Work out the finished part from the listing and answer in its coordinate system (mm). A direction names the side the tool comes from. Give positions to 0.01 mm unless a question says otherwise; leave off trailing zeros. Write each loop counter-clockwise with the first axis right and the second up, starting at its lowest first coordinate (ties: lowest second). Pieces come first, ordered by that corner, then holes.
1) Straight lines are drawn through the part: probe 1 along X at (y, z) = (38, 20.75); probe 2 along Y at (x, z) = (50, 20.45); probe 3 along X at (y, z) = (4, 27.5). For each, find the intervals that lie inside material, in ascending order.
2) Find section A-A (y = 57.5). Determine the outline of the cut face in (x, z).
3) A tool of negligible diameter and unlimited length cuts with its end or side. For faces 1 (the face through (49, 57, 27)), 2 (the face through (63, 57, 24)), 3 (the face through (53, 57, 28)), 4 (the face through (52, 18, 28)), from which of +Z, -Z, +X, -X, +Y, -Y can it reach the whole face along a straight path? Write none if from no direction.
4) Find section B-B (x = 125). Determine the outline of the cut face in (y, z), plus the area to 3 significant figures.
5) Find section C-C (y = 24). Determine the outline of the cut face in (x, z).
6) Determine the mould class of faces 5 (the face through (52, 44, 28)), 6 (the face through (50.74, 36.58, 20.48)), 7 (the face through (62, 18, 28)), 8 (the face through (126.11, 11.54, 19.49)) for opening direction X: pulls with the +X half, pulls with the -X half, needs draft (parallel to the pull), parting line crosses it, or undercut.
7) Given pin 1 Ø2.5 at (x, z) = (62, 22) entering from -Y; pin 2 Ø1.1 at (x, z) = (68.5, 26.5) entering from +Y; pin 3 Ø5 at (x, y) = (124, 33.5) entering from +Z, each flat-ended and moving along its own axis, determine where each tip first touches the part or whether it passes through.
8) Find section D-D (x = 135). Determine the outline of the cut face in (y, z).
```python
from build123d import *

# Parameters (mm, degrees)
CYLINDER455_R     = 1.2
CYLINDER455_DEPTH = 4
CYLINDER454_R     = 1.2
CYLINDER454_DEPTH = 4
BOX307_W          = 4
BOX307_H          = 6
BOX307_DEPTH      = 1
BOX308_W          = 10.5
BOX308_H          = 6
BOX308_DEPTH      = 1
BOX306_W          = 4
BOX306_H          = 6
BOX306_DEPTH      = 1
BOX305_W          = 75
BOX305_H          = 62
BOX305_DEPTH      = 1
BOX304_W          = 25
BOX304_H          = 62
BOX304_DEPTH      = 1
BOX303_W          = 25
BOX303_H          = 82
BOX303_DEPTH      = 2
BOX302_W          = 25
BOX302_H          = 82
BOX302_DEPTH      = 3
FILLET108_R       = 2.99
CYLINDER349_R     = 1.6
CYLINDER349_DEPTH = 10
CYLINDER351_R     = 1.6
CYLINDER351_DEPTH = 10
CYLINDER350_R     = 1.6
CYLINDER350_DEPTH = 10
CYLINDER347_R     = 1.6
CYLINDER347_DEPTH = 10
CYLINDER353_R     = 1.6
CYLINDER353_DEPTH = 10
BOX241_W          = 19
BOX241_H          = 5
BOX241_DEPTH      = 5
BOX242_W          = 4
BOX242_H          = 5
BOX242_DEPTH      = 8
BOX243_W          = 1.8
BOX243_H          = 7
BOX243_DEPTH      = 11
BOX244_W          = 8
BOX244_H          = 5
BOX244_DEPTH      = 8
BOX245_W          = 24
BOX245_H          = 10
BOX245_DEPTH      = 15
FILLET095_R       = 6
CYLINDER352_R     = 1.6
CYLINDER352_DEPTH = 10
BOX240_W          = 19
BOX240_H          = 5
BOX240_DEPTH      = 5
BOX239_W          = 4
BOX239_H          = 5
BOX239_DEPTH      = 8
BOX238_W          = 1.8
BOX238_H          = 7
BOX238_DEPTH      = 11
BOX236_W          = 8
BOX236_H          = 5
BOX236_DEPTH      = 8
BOX237_W          = 24
BOX237_H          = 10
BOX237_DEPTH      = 15
FILLET094_R       = 6
CYLINDER355_R     = 1.6
CYLINDER355_DEPTH = 10
BOX247_W          = 10
BOX247_H          = 10
BOX247_DEPTH      = 12
CYLINDER354_R     = 1.6
CYLINDER354_DEPTH = 10
BOX246_W          = 10
BOX246_H          = 10
BOX246_DEPTH      = 12
BOX235_W          = 24
BOX235_H          = 42
BOX235_DEPTH      = 3
FILLET109_R       = 6


with BuildPart() as cylinder455:
    # Cylinder455 → Cylinder455 (new body)
    with BuildSketch(Plane(origin=(125, 50, 15), x_dir=(1, 0, 0), z_dir=(0, 0, 1))):
        Circle(CYLINDER455_R)
    extrude(amount=CYLINDER455_DEPTH)


with BuildPart() as fusion409:
    # Cylinder454 → Cylinder454 (new body)
    with BuildSketch(Plane(origin=(125, 12, 15), x_dir=(1, 0, 0), z_dir=(0, 0, 1))):
        Circle(CYLINDER454_R)
    extrude(amount=CYLINDER454_DEPTH)

    # Fusion409: union Cylinder455
    add(cylinder455.part)


with BuildPart() as fusion409_1:
    # Fusion409 placement: moved
    add(fusion409.part.moved(Location((0, 0, 1))))


with BuildPart() as cube378:
    # Box307 → Box307 (new body)
    with BuildSketch(Plane(origin=(69, 54, 19), x_dir=(1, 0, 0), z_dir=(0, 0, 1))):
        with Locations((2, 3)):
            Rectangle(BOX307_W, BOX307_H)
    extrude(amount=BOX307_DEPTH)


with BuildPart() as cube379:
    # Box308 → Box308 (new body)
    with BuildSketch(Plane(origin=(133.5, 28, 19), x_dir=(1, 0, 0), z_dir=(0, 0, 1))):
        with Locations((5.25, 3)):
            Rectangle(BOX308_W, BOX308_H)
    extrude(amount=BOX308_DEPTH)


with BuildPart() as fusion410:
    # Box306 → Box306 (new body)
    with BuildSketch(Plane(origin=(69, 2, 19), x_dir=(1, 0, 0), z_dir=(0, 0, 1))):
        with Locations((2, 3)):
            Rectangle(BOX306_W, BOX306_H)
    extrude(amount=BOX306_DEPTH)

    # Fusion408: union Cube378, Cube379
    add(cube378.part)
    add(cube379.part)

    # Fusion410: union Fusion409
    add(fusion409_1.part)


with BuildPart() as cut303:
    # Box305 → Box305 (new body)
    with BuildSketch(Plane(origin=(69, 0, 19), x_dir=(1, 0, 0), z_dir=(0, 0, 1))):
        with Locations((37.5, 31)):
            Rectangle(BOX305_W, BOX305_H)
    extrude(amount=BOX305_DEPTH)

    # Cut303: cut Fusion410
    add(fusion410.part, mode=Mode.SUBTRACT)


with BuildPart() as cube375:
    # Box304 → Box304 (new body)
    with BuildSketch(Plane(origin=(45, 0, 19), x_dir=(1, 0, 0), z_dir=(0, 0, 1))):
        with Locations((12.5, 31)):
            Rectangle(BOX304_W, BOX304_H)
    extrude(amount=BOX304_DEPTH)


with BuildPart() as cube374:
    # Box303 → Box303 (new body)
    with BuildSketch(Plane(origin=(45, -10, 17), x_dir=(1, 0, 0), z_dir=(0, 0, 1))):
        with Locations((12.5, 41)):
            Rectangle(BOX303_W, BOX303_H)
    extrude(amount=BOX303_DEPTH)


with BuildPart() as fusion411:
    # Box302 → Box302 (new body)
    with BuildSketch(Plane(origin=(45, -10, 17), x_dir=(1, 0, 0), z_dir=(0, 0, 1))):
        with Locations((12.5, 41)):
            Rectangle(BOX302_W, BOX302_H)
    extrude(amount=BOX302_DEPTH)

    # Fillet108
    fillet108_edges = [fusion411.edges().sort_by_distance(p)[0] for p in [
        (57.5, -10, 20),
        (57.5, 72, 20),
    ]]
    fillet(fillet108_edges, radius=FILLET108_R)

    # Cut301: cut Cube374
    add(cube374.part, mode=Mode.SUBTRACT)

    # Cut302: cut Cube375
    add(cube375.part, mode=Mode.SUBTRACT)

    # Fusion411: union Cut303
    add(cut303.part)


with BuildPart() as cylinder349:
    # Cylinder349 → Cylinder349 (new body)
    with BuildSketch(Plane(origin=(50, 24, 12), x_dir=(1, 0, 0), z_dir=(0, 0, 1))):
        Circle(CYLINDER349_R)
    extrude(amount=CYLINDER349_DEPTH)


with BuildPart() as cylinder351:
    # Cylinder351 → Cylinder351 (new body)
    with BuildSketch(Plane(origin=(64, 24, 12), x_dir=(1, 0, 0), z_dir=(0, 0, 1))):
        Circle(CYLINDER351_R)
    extrude(amount=CYLINDER351_DEPTH)


with BuildPart() as cylinder350:
    # Cylinder350 → Cylinder350 (new body)
    with BuildSketch(Plane(origin=(64, 38, 12), x_dir=(1, 0, 0), z_dir=(0, 0, 1))):
        Circle(CYLINDER350_R)
    extrude(amount=CYLINDER350_DEPTH)


with BuildPart() as fusion300:
    # Cylinder347 → Cylinder347 (new body)
    with BuildSketch(Plane(origin=(50, 38, 12), x_dir=(1, 0, 0), z_dir=(0, 0, 1))):
        Circle(CYLINDER347_R)
    extrude(amount=CYLINDER347_DEPTH)

    # Fusion300: union Cylinder349, Cylinder351, Cylinder350
    add(cylinder349.part)
    add(cylinder351.part)
    add(cylinder350.part)


with BuildPart() as cylinder353:
    # Cylinder353 → Cylinder353 (new body)
    with BuildSketch(Plane(origin=(57, 52, 30), x_dir=(1, 0, 0), z_dir=(0, -1, 0))):
        Circle(CYLINDER353_R)
    extrude(amount=CYLINDER353_DEPTH)


with BuildPart() as cube321:
    # Box241 → Box241 (new body)
    with BuildSketch(Plane(origin=(54, 44.5, 19), x_dir=(1, 0, 0), z_dir=(0, 0, 1))):
        with Locations((9.5, 2.5)):
            Rectangle(BOX241_W, BOX241_H)
    extrude(amount=BOX241_DEPTH)


with BuildPart() as cube322:
    # Box242 → Box242 (new body)
    with BuildSketch(Plane(origin=(54, 44.5, 19), x_dir=(1, 0, 0), z_dir=(0, 0, 1))):
        with Locations((2, 2.5)):
            Rectangle(BOX242_W, BOX242_H)
    extrude(amount=BOX242_DEPTH)


with BuildPart() as cube323:
    # Box243 → Box243 (new body)
    with BuildSketch(Plane(origin=(53, 43.5, 19), x_dir=(1, 0, 0), z_dir=(0, 0, 1))):
        with Locations((0.9, 3.5)):
            Rectangle(BOX243_W, BOX243_H)
    extrude(amount=BOX243_DEPTH)


with BuildPart() as cube324:
    # Box244 → Box244 (new body)
    with BuildSketch(Plane(origin=(45, 44.5, 19), x_dir=(1, 0, 0), z_dir=(0, 0, 1))):
        with Locations((4, 2.5)):
            Rectangle(BOX244_W, BOX244_H)
    extrude(amount=BOX244_DEPTH)


with BuildPart() as fillet095:
    # Box245 → Box245 (new body)
    with BuildSketch(Plane(origin=(45, 42, 19), x_dir=(1, 0, 0), z_dir=(0, 0, 1))):
        with Locations((12, 5)):
            Rectangle(BOX245_W, BOX245_H)
    extrude(amount=BOX245_DEPTH)

    # Cut250: cut Cube324
    add(cube324.part, mode=Mode.SUBTRACT)

    # Cut254: cut Cube323
    add(cube323.part, mode=Mode.SUBTRACT)

    # Cut253: cut Cube322
    add(cube322.part, mode=Mode.SUBTRACT)

    # Cut251: cut Cube321
    add(cube321.part, mode=Mode.SUBTRACT)

    # Cut252: cut Cylinder353
    add(cylinder353.part, mode=Mode.SUBTRACT)

    # Fillet095
    fillet095_edges = [fillet095.edges().sort_by_distance(p)[0] for p in [
        (45, 47, 34),
        (69, 47, 34),
    ]]
    fillet(fillet095_edges, radius=FILLET095_R)


with BuildPart() as fillet095_1:
    # Fillet095 placement: moved
    add(fillet095.part.moved(Location((0, 10, 0))))


with BuildPart() as cylinder352:
    # Cylinder352 → Cylinder352 (new body)
    with BuildSketch(Plane(origin=(57, 52, 30), x_dir=(1, 0, 0), z_dir=(0, -1, 0))):
        Circle(CYLINDER352_R)
    extrude(amount=CYLINDER352_DEPTH)


with BuildPart() as cube320:
    # Box240 → Box240 (new body)
    with BuildSketch(Plane(origin=(54, 44.5, 19), x_dir=(1, 0, 0), z_dir=(0, 0, 1))):
        with Locations((9.5, 2.5)):
            Rectangle(BOX240_W, BOX240_H)
    extrude(amount=BOX240_DEPTH)


with BuildPart() as cube319:
    # Box239 → Box239 (new body)
    with BuildSketch(Plane(origin=(54, 44.5, 19), x_dir=(1, 0, 0), z_dir=(0, 0, 1))):
        with Locations((2, 2.5)):
            Rectangle(BOX239_W, BOX239_H)
    extrude(amount=BOX239_DEPTH)


with BuildPart() as cube318:
    # Box238 → Box238 (new body)
    with BuildSketch(Plane(origin=(53, 43.5, 19), x_dir=(1, 0, 0), z_dir=(0, 0, 1))):
        with Locations((0.9, 3.5)):
            Rectangle(BOX238_W, BOX238_H)
    extrude(amount=BOX238_DEPTH)


with BuildPart() as cube316:
    # Box236 → Box236 (new body)
    with BuildSketch(Plane(origin=(45, 44.5, 19), x_dir=(1, 0, 0), z_dir=(0, 0, 1))):
        with Locations((4, 2.5)):
            Rectangle(BOX236_W, BOX236_H)
    extrude(amount=BOX236_DEPTH)


with BuildPart() as fillet094:
    # Box237 → Box237 (new body)
    with BuildSketch(Plane(origin=(45, 42, 19), x_dir=(1, 0, 0), z_dir=(0, 0, 1))):
        with Locations((12, 5)):
            Rectangle(BOX237_W, BOX237_H)
    extrude(amount=BOX237_DEPTH)

    # Cut245: cut Cube316
    add(cube316.part, mode=Mode.SUBTRACT)

    # Cut246: cut Cube318
    add(cube318.part, mode=Mode.SUBTRACT)

    # Cut247: cut Cube319
    add(cube319.part, mode=Mode.SUBTRACT)

    # Cut248: cut Cube320
    add(cube320.part, mode=Mode.SUBTRACT)

    # Cut249: cut Cylinder352
    add(cylinder352.part, mode=Mode.SUBTRACT)

    # Fillet094
    fillet094_edges = [fillet094.edges().sort_by_distance(p)[0] for p in [
        (45, 47, 34),
        (69, 47, 34),
    ]]
    fillet(fillet094_edges, radius=FILLET094_R)


with BuildPart() as fillet094_1:
    # Fillet094 placement: moved
    add(fillet094.part.moved(Location((0, -42, 0))))


with BuildPart() as cylinder355:
    # Cylinder355 → Cylinder355 (new body)
    with BuildSketch(Plane(origin=(57, 52, 30), x_dir=(1, 0, 0), z_dir=(0, -1, 0))):
        Circle(CYLINDER355_R)
    extrude(amount=CYLINDER355_DEPTH)


with BuildPart() as cut256:
    # Box247 → Box247 (new body)
    with BuildSketch(Plane(origin=(52, 42, 22), x_dir=(1, 0, 0), z_dir=(0, 0, 1))):
        with Locations((5, 5)):
            Rectangle(BOX247_W, BOX247_H)
    extrude(amount=BOX247_DEPTH)

    # Cut256: cut Cylinder355
    add(cylinder355.part, mode=Mode.SUBTRACT)


with BuildPart() as cut256_1:
    # Cut256 placement: moved
    add(cut256.part.moved(Location((0, -32, 0))))


with BuildPart() as cylinder354:
    # Cylinder354 → Cylinder354 (new body)
    with BuildSketch(Plane(origin=(57, 52, 30), x_dir=(1, 0, 0), z_dir=(0, -1, 0))):
        Circle(CYLINDER354_R)
    extrude(amount=CYLINDER354_DEPTH)


with BuildPart() as cut255:
    # Box246 → Box246 (new body)
    with BuildSketch(Plane(origin=(52, 42, 22), x_dir=(1, 0, 0), z_dir=(0, 0, 1))):
        with Locations((5, 5)):
            Rectangle(BOX246_W, BOX246_H)
    extrude(amount=BOX246_DEPTH)

    # Cut255: cut Cylinder354
    add(cylinder354.part, mode=Mode.SUBTRACT)


with BuildPart() as fake_cylinder_holder_wide:
    # Box235 → Box235 (new body)
    with BuildSketch(Plane(origin=(45, 10, 19), x_dir=(1, 0, 0), z_dir=(0, 0, 1))):
        with Locations((12, 21)):
            Rectangle(BOX235_W, BOX235_H)
    extrude(amount=BOX235_DEPTH)

    # Fusion301: union Fillet095, Fillet094, Cut256, Cut255
    add(fillet095_1.part)
    add(fillet094_1.part)
    add(cut256_1.part)
    add(cut255.part)

    # Cut257: cut Fusion300
    add(fusion300.part, mode=Mode.SUBTRACT)

    # Fillet109
    fillet109_edges = [fake_cylinder_holder_wide.edges().sort_by_distance(p)[0] for p in [
        (62, 52, 28),
        (62, 10, 28),
        (52, 10, 28),
        (52, 52, 28),
    ]]
    fillet(fillet109_edges, radius=FILLET109_R)

    # Fusion412: union Fusion411
    add(fusion411.part)


solid = fake_cylinder_holder_wide.part
```
Results:
1. probe 1: x = 45 to 48.4, 51.6 to 62.4, 65.6 to 69
1. probe 2: y = 0 to 2.5, 7.5 to 22.4, 25.6 to 36.4, 39.6 to 54.5, 59.5 to 62
1. probe 3: x = 45 to 53, 54.8 to 69
2. outline: (45, 27) - (53, 27) - (53, 30) - (54.8, 30) - (54.8, 27) - (58, 27) - (58, 24) - (69, 24) - (69, 28) arc R6 ccw to (63, 34) - (51, 34) arc R6 ccw to (45, 28) - close; (73, 19) - (144, 19) - (144, 20) - (73, 20) - close; hole circle Ø3.2 at (57, 30)
3. face 1: -Z, -X
3. face 2: -Z, +X, -X
3. face 3: -Z
3. face 4: +Z, -X
4. outline: (0, 19) - (10.8, 19) - (10.8, 20) - (0, 20) - close; (13.2, 19) - (48.8, 19) - (48.8, 20) - (13.2, 20) - close; (51.2, 19) - (62, 19) - (62, 20) - (51.2, 20) - close
4. area: 57.2 mm2
5. outline: (45, 19) - (48.4, 19) - (48.4, 22) - (45, 22) - close; (51.6, 19) - (62.4, 19) - (62.4, 22) - (51.6, 22) - close; (65.6, 19) - (144, 19) - (144, 20) - (69, 20) - (69, 22) - (65.6, 22) - close
6. face 5: pulls with the -X half
6. face 6: undercut
6. face 7: pulls with the +X half
6. face 8: undercut
7. pin 1: stops at y = 0
7. pin 2: stops at y = 62
7. pin 3: stops at z = 20
8. outline: (0, 19) - (28, 19) - (28, 20) - (0, 20) - close; (34, 19) - (62, 19) - (62, 20) - (34, 20) - close
